Can you work these out from the model? Positions are in its coordinate system, mm. A direction names the side the tool comes from. Give positions to 0.01 mm unless a question says otherwise; leave off trailing zeros. Loops run counter-clockwise (first coordinate to the right, second up) from the corner with the lowest first, then second, coordinate; pieces in that order, holes last. Notation, with made-up numbers: M 39,62.25 L 62,62.25 A28 cw 62,96.25 Z; hole C 32.5,71.25 d1. An arc over 180 degrees is marked long. Answer as a JSON object with one key per item and string values.
Autodesk Inventor part; units mm, degrees
ref_plane "YZ Plane" through (0, 0, 0) normal (1, 0, 0) x (0, 1, 0)
ref_plane "XZ Plane" through (0, 0, 0) normal (0, 1, 0) x (-1, 0, 0)
ref_plane "XY Plane" through (0, 0, 0) normal (0, 0, 1) x (1, 0, 0)
sketch "Sketch1" plane through (0, 0, 0) normal (0, 0, 1) x (1, 0, 0)
  circle A0 centre (0, 0) radius 3
  dimension "Diameter" = 6
extrude "Extrusion1" add sketch "Sketch1" along normal blind 12.28
sketch "Sketch2" plane through (0, 0, 12.28) normal (0, 0, 1) x (1, 0, 0)
  circle A0 centre (0, 0) radius 3
extrude "Extrusion2" add sketch "Sketch2" along normal blind 3.72 draft 45
sketch "Sketch3" plane through (0, 0, 16) normal (0, 0, 1) x (1, 0, 0)
  circle A0 centre (0, 0) radius 6.72
  circle A1 centre (0, 0) radius 2.3094 construction
  line L0 (0.9667, 2.0973) -> (2.2997, 0.2115)
  line L1 (2.2997, 0.2115) -> (1.333, -1.8859)
  line L2 (1.333, -1.8859) -> (-0.9667, -2.0973)
  line L3 (-0.9667, -2.0973) -> (-2.2997, -0.2115)
  line L4 (-2.2997, -0.2115) -> (-1.333, 1.8859)
  line L5 (-1.333, 1.8859) -> (0.9667, 2.0973)
  dimension "Hex_Width" = 4
extrude "Extrusion3" cut sketch "Sketch3" against normal blind 2.5 contours L0 L1 L2 L3 L4 L5
thread "Thread1"
chamfer "Chamfer2" distance 0.6 angle 45 1 edges at (-3, 0, 0)
fillet "Fillet1" radius 0.1 1 edges at (-6.72, 0, 16)
equation "\"d10\" = Thread_Length"
equation "\"d13\" = Chamfer"
equation "\"Thread_Length\" = 12.28"
equation "\"Length\" = 16"
properties part number "SCREW,FLAT HD,P,12.9,M6X1.00X16MM"
1) Will these pins go through, and if not, where does the flat tip stop? pin 1 Ø1 at (y, z) = (0, 6.5) entering from -X; pin 2 Ø2 at (x, z) = (-5, 6) entering from -Y; pin 3 Ø2 at (x, y) = (0, -0.5) entering from +Z; pin 4 Ø1 at (x, y) = (3.5, 3) entering from -Z.
Answer list:
{"pin 1": "x = -3", "pin 2": "through", "pin 3": "z = 13.5", "pin 4": "z = 13.39"}
2) Suppose I cut it at B-B, the plane x = 0. Write out the boundary of the cut face in (y, z), and give its area (3 significant figures).
Answer list:
{"outline": "M -6.55,15.83 L -3,12.28 L -3,0.6 L -2.4,0 L 2.4,0 L 3,0.6 L 3,12.28 L 6.55,15.83 A0.1 ccw 6.48,16 L 2.01,16 L 2.01,13.5 L -2.01,13.5 L -2.01,16 L -6.48,16 A0.1 ccw Z", "area": "99.4 mm^2"}
3) Please list where these lines run through material, in increasing order: line 1 along Y through (x, z) = (1, 15); line 2 along Z through (x, y) = (1, -1.75); line 3 along Z through (x, y) = (-5.25, -2). Write a range as from..to.
Answer list:
{"line 1": "-5.63..-1.92, 2.05..5.63", "line 2": "0..13.5", "line 3": "14.9..16"}
4) Suppose I cut it at A-A, the plane z = 2. Write out the boundary of the cut face in (x, y), and give its area (3 significant figures).
Answer list:
{"outline": "C 0,0 d6", "area": "28.3 mm^2"}
5) Suppose I cut it at C-C, the plane y = 0. Write out the boundary of the cut face in (x, z).
Answer list:
{"outline": "M -6.55,15.83 L -3,12.28 L -3,0.6 L -2.4,0 L 2.4,0 L 3,0.6 L 3,12.28 L 6.55,15.83 A0.1 ccw 6.48,16 L 2.2,16 L 2.2,13.5 L -2.2,13.5 L -2.2,16 L -6.48,16 A0.1 ccw Z"}
6) If we mould it in two halves opening along Y, with no side actions, what happens to faces 4 (the conical face through (3.07, 0.97, 12.5)), 5 (the flat face through (0, 0, 0)), 6 (the flat face through (-1.823, 0.823, 14.768)), 7 (the flat face through (1.6, 1.2, 14.8))? For each: +Y half, -Y half, draft (parallel to the pull), parting line (faces both ways), or undercut.
Answer list:
{"face 4": "parting line", "face 5": "draft", "face 6": "undercut", "face 7": "undercut"}
7) For faces 1 (the flat face through (-2, -1, 16)), 2 (the flat face through (-1.6, -1.2, 14.8)), 3 (the cylindrical face through (-3, 0, 6)), which set-ups out of +Z, -Z, +X, -X, +Y, -Y let a thin tool reach every point of the face, with its end or its side?
Answer list:
{"face 1": "+Z, +X, -X, +Y, -Y", "face 2": "+Z", "face 3": "-Z"}
